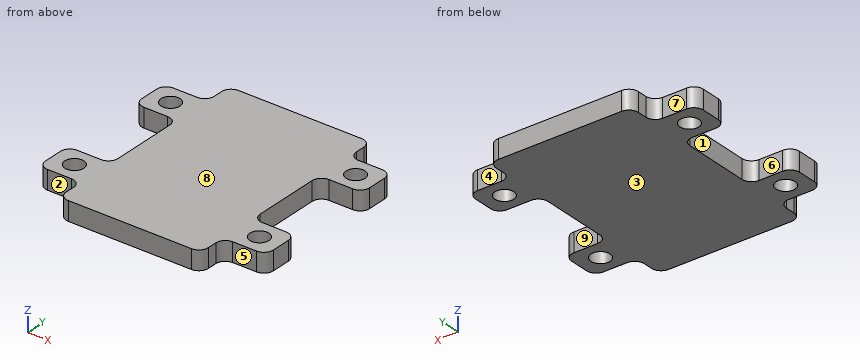
```python
from build123d import *

# Parameters (mm, degrees)
SKETCH1_R           = 0.5
BOSS_EXTRUDE1_DEPTH = 1


with BuildPart() as part:
    # Sketch1 → Boss-Extrude1 (new body)
    with BuildSketch(Plane.XY):
        with BuildLine():
            Line((-3.734024834, 11), (-3.734024834, 10.5))
            ThreePointArc((-3.734024834, 10.5), (-3.880471443, 10.146446609), (-4.234024834, 10))
            Line((-4.234024834, 10), (-5.484024834, 10))
            ThreePointArc((-5.484024834, 10), (-5.837578224, 9.853553391), (-5.984024834, 9.5))
            Line((-5.984024834, 9.5), (-5.984024834, 8.5))
            ThreePointArc((-5.984024834, 8.5), (-5.837578224, 8.146446609), (-5.484024834, 8))
            Line((-5.484024834, 8), (-4.234024834, 8))
            ThreePointArc((-4.234024834, 8), (-3.880471443, 7.853553391), (-3.734024834, 7.5))
            Line((-3.734024834, 7.5), (-3.734024834, 4))
            ThreePointArc((-3.734024834, 4), (-3.880471443, 3.646446609), (-4.234024834, 3.5))
            Line((-4.234024834, 3.5), (-5.484024834, 3.5))
            ThreePointArc((-5.484024834, 3.5), (-5.837578224, 3.353553391), (-5.984024834, 3))
            Line((-5.984024834, 3), (-5.984024834, 2))
            ThreePointArc((-5.984024834, 2), (-5.837578224, 1.646446609), (-5.484024834, 1.5))
            Line((-5.484024834, 1.5), (-4.234024834, 1.5))
            ThreePointArc((-4.234024834, 1.5), (-3.880471443, 1.353553391), (-3.734024834, 1))
            Line((-3.734024834, 1), (-3.734024834, 0.5))
            ThreePointArc((-3.734024834, 0.5), (-3.587578224, 0.146446609), (-3.234024834, 0))
            Line((-3.234024834, 0), (3.234024834, 0))
            ThreePointArc((3.234024834, 0), (3.587578224, 0.146446609), (3.734024834, 0.5))
            Line((3.734024834, 0.5), (3.734024834, 1))
            ThreePointArc((3.734024834, 1), (3.880471443, 1.353553391), (4.234024834, 1.5))
            Line((4.234024834, 1.5), (5.484024834, 1.5))
            ThreePointArc((5.484024834, 1.5), (5.837578224, 1.646446609), (5.984024834, 2))
            Line((5.984024834, 2), (5.984024834, 3))
            ThreePointArc((5.984024834, 3), (5.837578224, 3.353553391), (5.484024834, 3.5))
            Line((5.484024834, 3.5), (4.234024834, 3.5))
            ThreePointArc((4.234024834, 3.5), (3.880471443, 3.646446609), (3.734024834, 4))
            Line((3.734024834, 4), (3.734024834, 7.5))
            ThreePointArc((3.734024834, 7.5), (3.880471443, 7.853553391), (4.234024834, 8))
            Line((4.234024834, 8), (5.484024834, 8))
            ThreePointArc((5.484024834, 8), (5.837578224, 8.146446609), (5.984024834, 8.5))
            Line((5.984024834, 8.5), (5.984024834, 9.5))
            ThreePointArc((5.984024834, 9.5), (5.837578224, 9.853553391), (5.484024834, 10))
            Line((5.484024834, 10), (4.234024834, 10))
            ThreePointArc((4.234024834, 10), (3.880471443, 10.146446609), (3.734024834, 10.5))
            Line((3.734024834, 10.5), (3.734024834, 11))
            ThreePointArc((3.734024834, 11), (3.587578224, 11.353553391), (3.234024834, 11.5))
            Line((3.234024834, 11.5), (-3.234024834, 11.5))
            ThreePointArc((-3.234024834, 11.5), (-3.587578224, 11.353553391), (-3.734024834, 11))
        make_face()
        with Locations((-4.859024834, 9)):
            Circle(SKETCH1_R, mode=Mode.SUBTRACT)
        with Locations((-4.859024834, 2.5)):
            Circle(SKETCH1_R, mode=Mode.SUBTRACT)
        with Locations(Location((4.859024834, 2.5, 0), (0, 0, 180))):
            Circle(SKETCH1_R, mode=Mode.SUBTRACT)
        with Locations(Location((4.859024834, 9, 0), (0, 0, 180))):
            Circle(SKETCH1_R, mode=Mode.SUBTRACT)
    extrude(amount=BOSS_EXTRUDE1_DEPTH)


solid = part.part
```
Can you work these out from the model? Positions are in its coordinate system, mm. Face numbers are marked on the shaded views. A direction names the side the tool comes from. Coordinates: 2 decimals unless noted, no trailing zeros. Loops run counter-clockwise (first coordinate to the right, second up) from the corner with the lowest first, then second, coordinate; pieces in that order, holes last. Notation, with made-up numbers: (50, 28.5) - (67, 28.5) arc R26 ccw to (67, 53.5) - close; hole circle Ø4 at (36.5, 43.5). An arc over 180 degrees is marked (long way). Answer as CSV lines item,"result". Start each with the question number.
1) Suppose I cut it at C-C (y = 10.25). Please give me the cut outline in (x, z), plus the area to 3 significant figures.
2) For pin 1 (0.6 mm diameter, centred on y = 1, z = 0.5, fed in from -X); pin 2 (0.5 mm diameter, centred on y = 5.5, z = 0.5, fed in from -X); pin 3 (0.5 mm diameter, centred on x = -4.5, z = 0.5, fed in from -Y); pin 4 (5 mm diameter, centred on x = 4, y = 7.5, fed in from +Z), each with a flat end and sliding along its axis, tell me the tip position at first contact or that it passes through.
3) I need wall thicknesses on line 1 (Y direction, x = -4.75, z = 0.25); line 2 (X direction, y = 9.25, z = 0.7); line 3 (X direction, y = 6.25, z = 0.25). Which ranges of each line are inside material? Lowest first, please. Write a range as from..to.
4) Thinking about a two-plate mould opening in Y: for the marked faces 1, 2, 3 and 4, which applies, pulls with the +Y half, pulls with the -Y half, needs draft (parallel to the pull), parting line crosses it, or undercut?
5) Suppose I cut it at A-A (y = 2.5). Please give me the cut outline in (x, z), plus the area to 3 significant figures.
6) Which directions (+Z, -Z, +X, -X, +Y, -Y) give clear straight access to the entire face, cutting with the end or side of a thin tool? Please do the marked faces 5, 6, 7, 8 and 9.
7) Suppose I cut it at B-B (z = 0.8). Count the separate pieces of the cut face and the enclosed holes in it, plus the area to 3 significant figures.
Check result:
1,outline,"(-3.8, 0) - (3.8, 0) - (3.8, 1) - (-3.8, 1) - close"
1,area,"7.60 mm²"
2,pin 1,"stops at x = -3.83"
2,pin 2,"stops at x = -3.73"
2,pin 3,"stops at y = 1.5"
2,pin 4,"stops at z = 1"
3,line 1,"y = 1.5..2.01, 2.99..3.5, 8..8.51, 9.49..10"
3,line 2,"x = -5.98..-5.29, -4.43..4.43, 5.29..5.98"
3,line 3,"x = -3.73..3.73"
4,face 1,"undercut"
4,face 2,"pulls with the -Y half"
4,face 3,"needs draft"
4,face 4,"pulls with the +Y half"
5,outline,"(-5.98, 0) - (-5.36, 0) - (-5.36, 1) - (-5.98, 1) - close; (-4.36, 0) - (4.36, 0) - (4.36, 1) - (-4.36, 1) - close; (5.36, 0) - (5.98, 0) - (5.98, 1) - (5.36, 1) - close"
5,area,"9.97 mm²"
6,face 5,"+Z, -Z, +X, -Y"
6,face 6,"+Z, -Z, -X"
6,face 7,"+Z, -Z, -X, +Y"
6,face 8,"+Z, +X, -X, +Y, -Y"
6,face 9,"+Z, -Z, +X"
7,separate pieces,"1"
7,enclosed holes,"4"
7,area,"101 mm²"
